Here's the drawing with two shaded views (mm, measured from the low corner). I have some questions. A direction names the side the tool comes from. Coordinates: 2 decimals unless noted, no trailing zeros. Loops run counter-clockwise (first coordinate to the right, second up) from the corner with the lowest first, then second, coordinate; pieces in that order, holes last. Notation, with made-up numbers: M 27.25,20 L 42.25,20 A18 cw 42.25,51 Z; hole C -22,-26 d7. An arc over 180 degrees is marked long. Return JSON: item names as keys, results as strings. Group by question number.
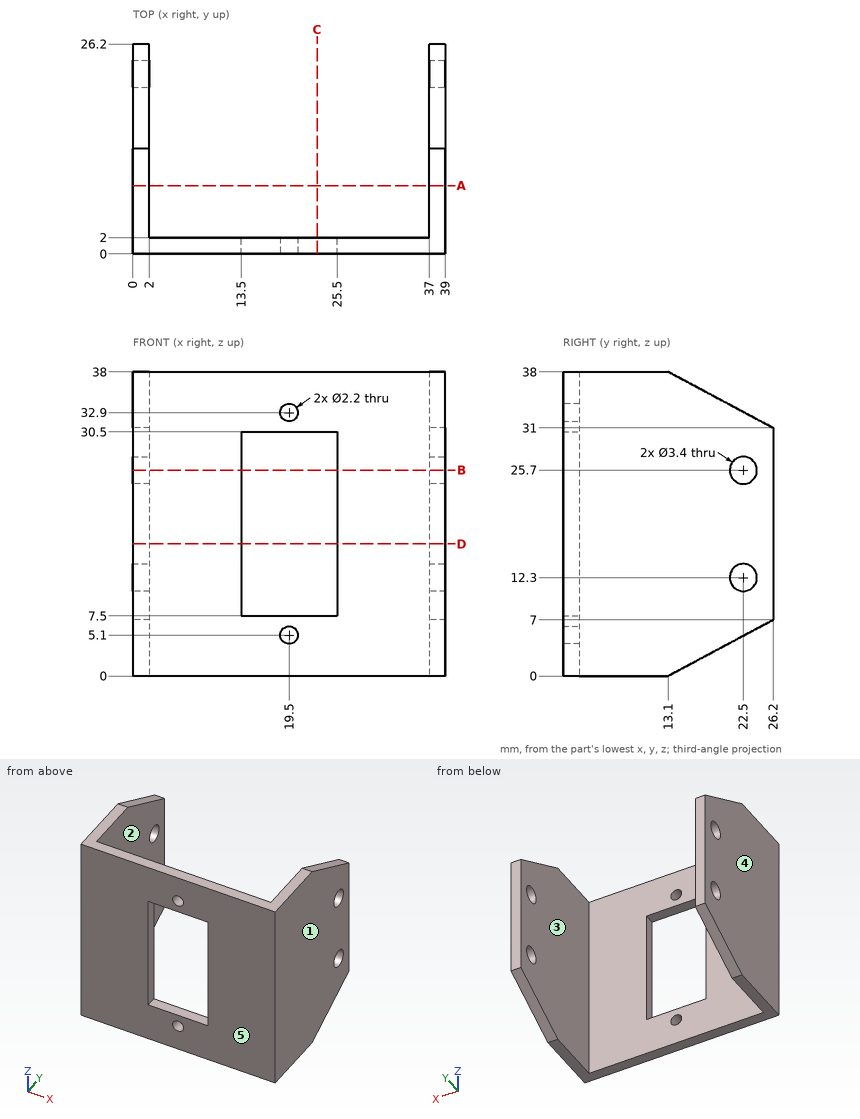
(1) Imagine slicing it at C-C, the plane x = 23. Write out the boundary of the cut face in (y, z).
(2) If I drill on L1, parallel to X at y = 0.7, z = 5.1; L2, parallel to X at y = 12, z = 15; L3, parallel to Y at x = 10, z = 31, over which ranges is the centre line in solid material (lowest first)? Write a range as [from, to].
(3) Imagine slicing it at B-B, the plane z = 25.7. Write out the boundary of the cut face in (x, y), then the cut area to 3 significant figures.
(4) We'd pull the mould along X, two halves only. Please class the marked faces 3, 4 and 5: +X half, -X half, draft (parallel to the pull), parting line (faces both ways), or undercut.
(5) Imagine slicing it at D-D, the plane z = 16.5. Write out the boundary of the cut face in (x, y), then the cut area to 3 significant figures.
(6) For the marked faces 1 and 2, which set-ups out of +Z, -Z, +X, -X, +Y, -Y let a thin tool reach every point of the face, with its end or its side?
(7) Imagine slicing it at A-A, the plane y = 8.5. Write out the boundary of the cut face in (x, z), then the cut area to 3 significant figures.
(8) Will this pin go through, and if not, where does the flat tip stop? P1, Ø10.5, axis at x = 17, z = 19.5, coming from the +Y side.
Checks:
{
 "1": {"outline": "M 0,0 L 2,0 L 2,7.5 L 0,7.5 Z; M 0,30.5 L 2,30.5 L 2,38 L 0,38 Z"},
 "2": {"L1": "[0, 18.4], [20.6, 39]", "L2": "[0, 2], [37, 39]", "L3": "[0, 2]"},
 "3": {"outline": "M 0,0 L 13.5,0 L 13.5,2 L 2,2 L 2,20.8 L 0,20.8 Z; M 0,24.2 L 2,24.2 L 2,26.2 L 0,26.2 Z; M 25.5,0 L 39,0 L 39,20.8 L 37,20.8 L 37,2 L 25.5,2 Z; M 37,24.2 L 39,24.2 L 39,26.2 L 37,26.2 Z", "area": "137 mm²"},
 "4": {"face 3": "undercut", "face 4": "-X half", "face 5": "draft"},
 "5": {"outline": "M 0,0 L 13.5,0 L 13.5,2 L 2,2 L 2,26.2 L 0,26.2 Z; M 25.5,0 L 39,0 L 39,26.2 L 37,26.2 L 37,2 L 25.5,2 Z", "area": "151 mm²"},
 "6": {"face 1": "+Z, -Z, +X, +Y, -Y", "face 2": "+Z, -Z, +Y"},
 "7": {"outline": "M 0,0 L 2,0 L 2,38 L 0,38 Z; M 37,0 L 39,0 L 39,38 L 37,38 Z", "area": "152 mm²"},
 "8": {"P1": "y = 2"}
}
